```python
from build123d import *

# Parameters (mm, degrees)
BOSS_EXTRUDE1_START     = 6
BOSS_EXTRUDE1_DEPTH     = 12
BOSS_EXTRUDE2_START     = -6
BOSS_EXTRUDE2_DEPTH     = 12
SKETCH3_R               = 22.5
BOSS_EXTRUDE3_DEPTH     = 25
HOLE1_D                 = 18
HOLE2_D                 = 18
HOLE3_D                 = 10
FILLET1_R               = 10
CUT_EXTRUDE1_DEPTH      = 95.757585448
CUT_EXTRUDE1_DEPTH_BACK = 95.757585448
SKETCH11_R              = 22.5


with BuildPart() as part:
    # Sketch1 → Boss-Extrude1 (new body)
    with BuildSketch(Plane(origin=(0, 0, 0), x_dir=(0, 0, -1), z_dir=(1, 0, 0)).offset(BOSS_EXTRUDE1_START)):
        with BuildLine():
            Line((18, 55), (18, -55))
            ThreePointArc((18, -55), (0, -73), (-18, -55))
            Line((-18, -55), (-18, 55))
            ThreePointArc((-18, 55), (0, 73), (18, 55))
        make_face()
    extrude(amount=BOSS_EXTRUDE1_DEPTH)



with BuildPart() as body_2:
    # Sketch2 → Boss-Extrude2 (new body)
    with BuildSketch(Plane(origin=(0, 0, 0), x_dir=(0, 0, -1), z_dir=(1, 0, 0)).offset(BOSS_EXTRUDE2_START)):
        with BuildLine():
            Line((18, -55), (18, 55))
            ThreePointArc((18, 55), (0, 73), (-18, 55))
            Line((-18, 55), (-18, -55))
            ThreePointArc((-18, -55), (0, -73), (18, -55))
        make_face()
    extrude(amount=-BOSS_EXTRUDE2_DEPTH)


with BuildPart() as part_1:
    add(part.part)

    add(body_2.part)  # Boss-Extrude3 merges body 2
    # Sketch3 → Boss-Extrude3 (add, symmetric)
    with BuildSketch(Plane.XY):
        with BuildLine():
            Line((-35, 9), (-28.618176043, 9))
            ThreePointArc((-28.618176043, 9), (-1.060743162, 29.981241201), (27.910571474, 11))
            Line((27.910571474, 11), (55, 11))
            Line((55, 11), (55, 3))
            Line((55, 3), (29.849623113, 3))
            ThreePointArc((29.849623113, 3), (30, 0), (29.849623113, -3))
            Line((29.849623113, -3), (55, -3))
            Line((55, -3), (55, -11))
            Line((55, -11), (27.910571474, -11))
            ThreePointArc((27.910571474, -11), (-1.060743162, -29.981241201), (-28.618176043, -9))
            Line((-28.618176043, -9), (-35, -9))
            Line((-35, -9), (-35, 9))
        make_face()
        Circle(SKETCH3_R, mode=Mode.SUBTRACT)
    extrude(amount=BOSS_EXTRUDE3_DEPTH, both=True)

    # Hole1 (through all)
    with Locations(Plane(origin=(18, 0, 0), x_dir=(0, 0, -1), z_dir=(1, 0, 0))):
        with Locations((0, 55)):
            Hole(HOLE1_D / 2)

    # Hole2 (through all)
    with Locations(Plane(origin=(18, 0, 0), x_dir=(0, 0, -1), z_dir=(1, 0, 0))):
        with Locations((0, -55)):
            Hole(HOLE2_D / 2)

    # Hole3 (through all)
    with Locations(Plane(origin=(0, 11, 0), x_dir=(1, 0, 0), z_dir=(0, 1, 0))):
        with Locations((43, -13)):
            hole3 = Hole(HOLE3_D / 2)

    # Mirror2: Hole3 across plane
    add(hole3.mirror(Plane.XY), mode=Mode.SUBTRACT)

    # Fillet1
    fillet1_edges = [part_1.edges().sort_by_distance(p)[0] for p in [
        (55, -7, 25),
        (55, 7, 25),
        (55, -7, -25),
        (55, 7, -25),
    ]]
    fillet(fillet1_edges, radius=FILLET1_R)

    # Sketch11 → Cut-Extrude1 (cut, two sides: drawn at the far end of the back side and taken through both)
    with BuildSketch(Plane.XY.offset(-CUT_EXTRUDE1_DEPTH_BACK)):
        Circle(SKETCH11_R)
    extrude(amount=CUT_EXTRUDE1_DEPTH + CUT_EXTRUDE1_DEPTH_BACK, mode=Mode.SUBTRACT)


solid = part_1.part
```
CAD build for the part. Positions are in the model's coordinates, mm. A direction names the side the tool comes from. Coordinates: 2 decimals unless noted, no trailing zeros. Order: outer loops, then holes, each group sorted by start corner. A loop starts at its lowest first (then second) coordinate and runs counter-clockwise, first axis right, second up.
(1) Pin check, flat tips, straight feed: pin 1 Ø13 at (x, y) = (-11, 45) entering from -Z; pin 2 Ø2 at (x, z) = (24.5, 15.5) entering from -Y; pin 3 Ø1.9 at (x, z) = (-32.5, -8) entering from -Y. Stop position of each tip, or through.
Solution:
pin 1: stops at z = -18
pin 2: stops at y = -18.65
pin 3: stops at y = -9
(2) Drill centre lines: L1, parallel to Z at x = 43, y = 8; L2, parallel to X at y = -48, z = -12.5; L3, parallel to Y at x = -14.5, z = -8. Where is each one in solid material? Low to high.
Solution:
L1: z = -25 to -18, -8 to 8, 18 to 25
L2: x = -18 to -6, 6 to 18
L3: y = -71.12 to -59.12, -50.88 to -17.2, 17.2 to 50.88, 59.12 to 71.12
(3) Saw through at D-D, the plane y = 56.5. Write the cut outline in (x, z), and give its area (3 significant figures).
Solution:
outline: (-18, -17.94) - (-6, -17.94) - (-6, -8.87) - (-18, -8.87) - close; (-18, 8.87) - (-6, 8.87) - (-6, 17.94) - (-18, 17.94) - close; (6, -17.94) - (18, -17.94) - (18, -8.87) - (6, -8.87) - close; (6, 8.87) - (18, 8.87) - (18, 17.94) - (6, 17.94) - close
area: 435 mm2
(4) Saw through at A-A, the plane x = 43. Write the cut outline in (y, z), and give its area (3 significant figures).
Solution:
outline: (-11, -25) - (-3, -25) - (-3, -18) - (-11, -18) - close; (-11, -8) - (-3, -8) - (-3, 8) - (-11, 8) - close; (-11, 18) - (-3, 18) - (-3, 25) - (-11, 25) - close; (3, -25) - (11, -25) - (11, -18) - (3, -18) - close; (3, -8) - (11, -8) - (11, 8) - (3, 8) - close; (3, 18) - (11, 18) - (11, 25) - (3, 25) - close
area: 480 mm2
(5) Mould opens along Y. For faces 5 (the face through (10.382, -19.961, -0.35)), 6 (the face through (-32, 9, 0)), 7 (the face through (12, -40, 18)) say: released by +Y, released by -Y, zero draft, split by the parting line, or undercut.
Solution:
face 5: undercut
face 6: released by +Y
face 7: zero draft
(6) Saw through at B-B, the plane y = 0. Write the cut outline in (x, z), and give its area (3 significant figures).
Solution:
outline: (-35, -25) - (-22.5, -25) - (-22.5, 25) - (-35, 25) - close; (22.5, -25) - (30, -25) - (30, 25) - (22.5, 25) - close
area: 1,000 mm2
(7) Saw through at C-C, the plane x = -11.5. Write the cut outline in (y, z), and give its area (3 significant figures).
Solution:
outline: (-55, -18) - (-27.71, -18) - (-27.71, -25) - (-19.34, -25) - (-19.34, 25) - (-27.71, 25) - (-27.71, 18) - (-55, 18) arc R18 ccw to start; (19.34, -25) - (27.71, -25) - (27.71, -18) - (55, -18) arc R18 ccw to (55, 18) - (27.71, 18) - (27.71, 25) - (19.34, 25) - close; hole circle Ø18 at (-55, 0); hole circle Ø18 at (55, 0)
area: 3,310 mm2
(8) Which spindle directions (+Z, -Z, +X, -X, +Y, -Y) get a long thin tool onto all of the face, cutting with end or side? Do faces 1 (the face through (-12, 39, -18)), 2 (the face through (-12, 40, 18)), 3 (the face through (-12, -40, -18)), 4 (the face through (6, 46.7, -4.3)). Say none if no direction does.
Solution:
face 1: -Z, -X, +Y
face 2: +Z, -X, +Y
face 3: -Z, -X, -Y
face 4: +Z, -Z, +Y
